Input: part model. Units: mm. Frame: model coordinates. Face numbers are marked on the shaded views. A direction names the side the tool comes from. Give positions to 0.01 mm unless a question says otherwise; leave off trailing zeros. Loops run counter-clockwise (first coordinate to the right, second up) from the corner with the lowest first, then second, coordinate; pieces in that order, holes last.
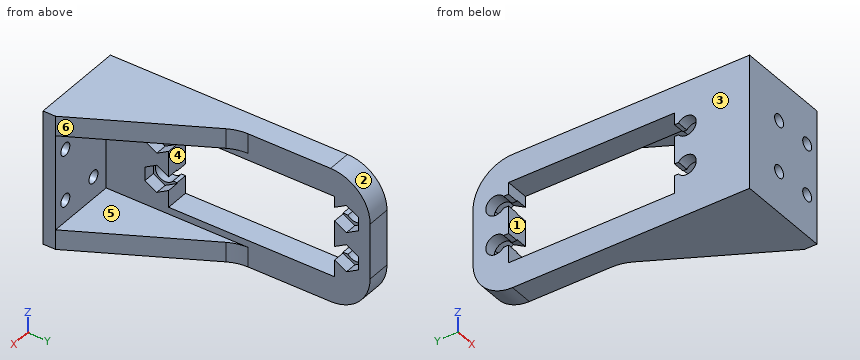
from build123d import *

# Parameters (mm, degrees)
SKETCH1_W                    = 34
SKETCH1_H                    = 70
SKETCH1_W_2                  = 20.5
SKETCH1_H_2                  = 42
BOSS_EXTRUDE1_DEPTH          = 3
CUT_EXTRUDE1_DEPTH           = 45.170833137
CUT_EXTRUDE2_DEPTH           = 3
SKETCH4_W                    = 24
SKETCH4_H                    = 34
BOSS_EXTRUDE2_DEPTH          = 3.175
BOSS_EXTRUDE3_DEPTH          = 5
BOSS_EXTRUDE4_DEPTH          = 5
F_1_8_0_125_DIAMETER_HOLE1_D = 3.175
FILLET1_R                    = 10
FILLET2_R                    = 10


with BuildPart() as part:
    # Sketch1 → Boss-Extrude1 (new, symmetric)
    with BuildSketch(Plane(origin=(0, 0, 0), x_dir=(0, 0, -1), z_dir=(1, 0, 0))):
        with Locations((0.75, -5)):
            Rectangle(SKETCH1_W, SKETCH1_H)
        with Locations((0.75, 0)):
            Rectangle(SKETCH1_W_2, SKETCH1_H_2, mode=Mode.SUBTRACT)
    extrude(amount=BOSS_EXTRUDE1_DEPTH, both=True)

    # Sketch2 → Cut-Extrude1 (cut, through all)
    with BuildSketch(Plane.ZY.offset(3)):
        with BuildLine():
            Line((3.5, -21), (6.5, -21))
            Line((6.5, -21), (6.5, -22))
            ThreePointArc((6.5, -22), (5, -26.5), (3.5, -22))
            Line((3.5, -22), (3.5, -21))
        make_face()
        with BuildLine():
            Line((-6.5, -21), (-3.5, -21))
            Line((-3.5, -21), (-3.5, -22))
            ThreePointArc((-3.5, -22), (-5, -26.5), (-6.5, -22))
            Line((-6.5, -22), (-6.5, -21))
        make_face()
        with BuildLine():
            Line((6.5, 21), (6.5, 22.26))
            ThreePointArc((6.5, 22.26), (5, 26.76), (3.5, 22.26))
            Line((3.5, 22.26), (3.5, 21))
            Line((3.5, 21), (6.5, 21))
        make_face()
        with BuildLine():
            Line((-3.5, 21), (-3.5, 22.26))
            ThreePointArc((-3.5, 22.26), (-5, 26.76), (-6.5, 22.26))
            Line((-6.5, 22.26), (-6.5, 21))
            Line((-6.5, 21), (-3.5, 21))
        make_face()
    extrude(amount=-CUT_EXTRUDE1_DEPTH, mode=Mode.SUBTRACT)

    # Sketch3 → Cut-Extrude2 (cut)
    with BuildSketch(Plane(origin=(3, 0, 0), x_dir=(0, 0, -1), z_dir=(1, 0, 0))):
        Polygon((-3.267949192, 27), (-6.732050808, 27), (-8.464101615, 24), (-6.732050808, 21), (-3.267949192, 21), (-1.535898385, 24), align=None)
        Polygon((1.535898385, 24), (3.267949192, 27), (6.732050808, 27), (8.464101615, 24), (6.732050808, 21), (3.267949192, 21), align=None)
        Polygon((3.267949192, -27), (6.732050808, -27), (8.464101615, -24), (6.732050808, -21), (3.267949192, -21), (1.535898385, -24), align=None)
        Polygon((-1.535898385, -24), (-3.267949192, -27), (-6.732050808, -27), (-8.464101615, -24), (-6.732050808, -21), (-3.267949192, -21), align=None)
    extrude(amount=-CUT_EXTRUDE2_DEPTH, mode=Mode.SUBTRACT)

    # Sketch4 → Boss-Extrude2 (add)
    with BuildSketch(Plane.XZ.offset(40)):
        with Locations((9, -0.75)):
            Rectangle(SKETCH4_W, SKETCH4_H)
    extrude(amount=-BOSS_EXTRUDE2_DEPTH)

    # Sketch5 → Boss-Extrude3 (add)
    with BuildSketch(Plane(origin=(0, 0, -17.75), x_dir=(-1, 0, 0), z_dir=(0, 0, -1))):
        Polygon((-3, -36.825), (-21, -36.825), (-3, -3.4125), align=None)
    extrude(amount=-BOSS_EXTRUDE3_DEPTH)

    # Sketch6 → Boss-Extrude4 (add)
    with BuildSketch(Plane.XY.offset(16.25)):
        Polygon((21, -36.825), (3, -36.825), (3, -3.4125), align=None)
    extrude(amount=-BOSS_EXTRUDE4_DEPTH)

    # 1_8 _0.125_ Diameter Hole1 (through all)
    with Locations(Plane(origin=(0, -36.825, 0), x_dir=(1, 0, 0), z_dir=(0, 1, 0))):
        with Locations((7.5, 7.25), (17.5, 7.25), (17.5, -5.75), (7.5, -5.75)):
            Hole(F_1_8_0_125_DIAMETER_HOLE1_D / 2)

    # Fillet1
    fillet1_edges = [part.edges().sort_by_distance(p)[0] for p in [
        (0, 30, 16.25),
        (0, 30, -17.75),
    ]]
    fillet(fillet1_edges, radius=FILLET1_R)

    # Fillet2
    fillet2_edges = [part.edges().sort_by_distance(p)[0] for p in [
        (3, -3.4125, -15.25),
        (3, -3.4125, 13.75),
    ]]
    fillet(fillet2_edges, radius=FILLET2_R)


solid = part.part
(1) Cut plane D-D (z = 5). Return the cut outline in (x, y) (3 decimals), and give its area (3 significant figures).
Values follow:
outline: (-3, -40) - (6.101, -40) - (6.101, -36.825) - (3, -36.825) - (3, -27) - (0, -27) - (0, -26.5) - (-3, -26.5) - close; (-3, 26.76) - (0, 26.76) - (0, 27) - (3, 27) - (3, 30) - (-3, 30) - close; (8.899, -40) - (16.101, -40) - (16.101, -36.825) - (8.899, -36.825) - close; (18.899, -40) - (21, -40) - (21, -36.825) - (18.899, -36.825) - close
area: 138 mm2
(2) Cut plane A-A (y = 17). Return the cut outline in (x, z).
Values follow:
outline: (-3, -17.75) - (3, -17.75) - (3, -11) - (-3, -11) - close; (-3, 9.5) - (3, 9.5) - (3, 16.25) - (-3, 16.25) - close
(3) Ray query, probe 1 along Z at (x, y) = (-1.4, -24); probe 2 along X at (y, z) = (-38.1, -7.25); probe 3 along Z at (x, y) = (5.5, -28). Return the intervals inside material, ascending.
Values follow:
probe 1: z = -17.75 to -7.5, -2.5 to 2.5, 7.5 to 16.25
probe 2: x = -3 to 5.91, 9.09 to 15.91, 19.09 to 21
probe 3: z = -17.75 to -12.75, 11.25 to 16.25
(4) Cut plane C-C (x = 17.5). Count the separate pieces of the cut face and the enclosed holes in it, and give its area (3 significant figures).
Values follow:
separate pieces: 3
enclosed holes: 0
area: 153 mm2
(5) Cut plane B-B (z = -5). Return the cut outline in (x, y) (3 decimals).
Values follow:
outline: (-3, -40) - (21, -40) - (21, -36.825) - (3, -36.825) - (3, -27) - (0, -27) - (0, -26.5) - (-3, -26.5) - close; (-3, 26.76) - (0, 26.76) - (0, 27) - (3, 27) - (3, 30) - (-3, 30) - close
(6) Mould query, pull axis Z, two halves, no side actions, for the marked faces 1, 2 and 3. Classes: +Z half, -Z half, draft (parallel to the pull), parting line (faces both ways), or undercut.
Values follow:
face 1: undercut
face 2: +Z half
face 3: draft
(7) Pin query (flat end, axial travel): pin 1 Ø1.5 at (x, z) = (0.5, 7.5) entering from +Y; pin 2 Ø9 at (x, z) = (14, -3.5) entering from +Y (3 decimals); pin 3 Ø1.4 at (x, y) = (-1.5, 22) entering from +Z. Return the tip coordinate at first contact, or that it passes through.
Values follow:
pin 1: stops at y = 29.99
pin 2: stops at y = -36.825
pin 3: stops at z = 16.17
(8) Reachability of the marked faces 4, 5 and 6 from +Z, -Z, +X, -X, +Y, -Y: full face, straight path, thin tool, end or side. Return the list, or none.
Values follow:
face 4: +X, -X
face 5: +X, +Y
face 6: +Z, -Z, +X, +Y
